from build123d import *

# Parameters (mm, degrees)
SKETCH1_R           = 25.4
BOSS_EXTRUDE1_DEPTH = 1.5875
SKETCH2_R           = 1.524
CUT_EXTRUDE1_DEPTH  = 2.5875
CIRPATTERN1_COUNT   = 4


with BuildPart() as part:
    # Sketch1 → Boss-Extrude1 (new body)
    with BuildSketch(Plane.XY):
        Circle(SKETCH1_R)
    extrude(amount=BOSS_EXTRUDE1_DEPTH)

    # Sketch2 → Cut-Extrude1 (cut, through all)
    with BuildSketch(Plane.XY.offset(1.5875)):
        with Locations((0, 22.225)):
            Circle(SKETCH2_R)
    cut_extrude1 = extrude(amount=-CUT_EXTRUDE1_DEPTH, mode=Mode.SUBTRACT)

    # CirPattern1: Cut-Extrude1 ×4 about axis
    cirpattern1_axis = Axis((0, 0, 0), (0, 0, 1))
    for i in range(1, CIRPATTERN1_COUNT):
        add(cut_extrude1.rotate(cirpattern1_axis, i * 360 / CIRPATTERN1_COUNT), mode=Mode.SUBTRACT)


solid = part.part
Design review of the part built by this model. Coordinates are the model's own, in mm. Coordinates: 2 decimals unless noted, no trailing zeros. Write each loop counter-clockwise with the first axis right and the second up, starting at its lowest first coordinate (ties: lowest second). Pieces come first, ordered by that corner, then holes. Notation, with made-up numbers: (15.25, 7) -> (33.25, 7) arc R20 ccw to (33.25, 28) -> close; hole circle Ø8 at (-38.5, -2). An arc over 180 degrees is marked (long way). Write each question's results on one line, items separated by ' | '. Start each with the question number.
(1) Take a section at C-C on z = 0.3. Write out the cut boundary in (x, y) (3 decimals), and give its area (3 significant figures).
(2) The part is to be moulded in two halves that separate along Y. For faces 1 (the face through (0, 0, 1.588)), 2 (the face through (-0.33, 20.737, 0.805)), 3 (the face through (-5.506, -24.796, 0.783)), say which applies: pulls with the +Y half, pulls with the -Y half, needs draft (parallel to the pull), parting line crosses it, or undercut.
(3) Take a section at D-D on y = 17. Write out the cut boundary in (x, z).
(4) For line 1 along Y through (x, z) = (0, 1.05); line 2 along Y through (x, z) = (21, 0.65); line 3 along Y through (x, z) = (9, 1.15), list the stretches that pass through material, from the lowest coordinate up. Write a range as from..to.
(5) Take a section at A-A on y = 0. Write out the cut boundary in (x, z).
Results found:
1) outline: circle Ø50.8 at (0, 0); hole circle Ø3.048 at (-22.225, 0); hole circle Ø3.048 at (0, -22.225); hole circle Ø3.048 at (0, 22.225); hole circle Ø3.048 at (22.225, 0) | area: 2,000 mm2
2) face 1: needs draft | face 2: undercut | face 3: parting line crosses it
3) outline: (-18.87, 0) -> (18.87, 0) -> (18.87, 1.59) -> (-18.87, 1.59) -> close
4) line 1: y = -25.4..-23.75, -20.7..20.7, 23.75..25.4 | line 2: y = -14.29..-0.91, 0.91..14.29 | line 3: y = -23.75..23.75
5) outline: (-25.4, 0) -> (-23.75, 0) -> (-23.75, 1.59) -> (-25.4, 1.59) -> close; (-20.7, 0) -> (20.7, 0) -> (20.7, 1.59) -> (-20.7, 1.59) -> close; (23.75, 0) -> (25.4, 0) -> (25.4, 1.59) -> (23.75, 1.59) -> close
